from build123d import *

# Parameters (mm, degrees)
SKETCH_1_W                  = 28
SKETCH_1_H                  = 19
EXTRUDE_1_DEPTH             = 29
CUT_EXTRUDE_1_DEPTH         = 42.41557678
HOLE_WIZARD_1_D             = 10
HOLE_WIZARD_1_2_D           = 5.5
HOLE_WIZARD_1_2_CBORE_D     = 10
HOLE_WIZARD_1_2_CBORE_DEPTH = 5
CHAMFER_1_SIZE              = 5


with BuildPart() as part:
    # 草图1 → 凸台-拉伸1 (new body)
    with BuildSketch(Plane(origin=(0, 0, 0), x_dir=(1, 0, 0), z_dir=(0, 1, 0))):
        Rectangle(SKETCH_1_W, SKETCH_1_H)
    extrude(amount=-EXTRUDE_1_DEPTH)

    # 草图2 → 切除-拉伸1 (cut, through all)
    with BuildSketch(Plane(origin=(14, 0, 0), x_dir=(0, 0, -1), z_dir=(1, 0, 0))):
        with BuildLine():
            Line((9.5, -29), (-5, -29))
            Line((-5, -29), (-5, -10))
            ThreePointArc((-5, -10), (-4.121320344, -7.878679656), (-2, -7))
            Line((-2, -7), (9.5, -7))
            Line((9.5, -7), (9.5, -29))
        make_face()
    extrude(amount=-CUT_EXTRUDE_1_DEPTH, mode=Mode.SUBTRACT)

    # Hole Wizard 1 (through all)
    with Locations(Plane.XY.offset(9.5)):
        with Locations((0, -19)):
            Hole(HOLE_WIZARD_1_D / 2)

    # Hole Wizard 1 2 (through all)
    with Locations(Plane(origin=(0, -7, 0), x_dir=(-1, 0, 0), z_dir=(0, -1, 0))):
        with Locations((8, 3.5), (-8, 3.5)):
            CounterBoreHole(HOLE_WIZARD_1_2_D / 2, HOLE_WIZARD_1_2_CBORE_D / 2, HOLE_WIZARD_1_2_CBORE_DEPTH)

    # 倒角1
    chamfer_1_edges = [part.edges().sort_by_distance(p)[0] for p in [
        (-14, -29, 7.25),
        (14, -29, 7.25),
    ]]
    chamfer(chamfer_1_edges, length=CHAMFER_1_SIZE)


solid = part.part
Verification items for the finished model (mm, model axes). A direction names the side the tool comes from. Coordinates: 2 decimals unless noted, no trailing zeros. Order: outer loops, then holes, each group sorted by start corner. A loop starts at its lowest first (then second) coordinate and runs counter-clockwise, first axis right, second up. Notation, with made-up numbers: (17, 21) -> (41, 21) arc R20 ccw to (41, 31) -> close; hole circle Ø2 at (12.25, 9.25). An arc over 180 degrees is marked (long way). Put each result on its own line as item: value. Start each with the question number.
1. Material ranges on L1, parallel to Y at x = 0, z = 6.8; L2, parallel to X at y = -2.25, z = -8; L3, parallel to Z at x = -8, y = -4.65, recorded low to high. Write a range as [from, to].
2. Mould release check, pull along Z, two halves, no side actions. Record for faces 1 (the flat face through (0, -11, 9.5)), 2 (the flat face through (-11, -27, 7)), 3 (the cylindrical face through (-6.73, -0.99, -1.06)): released by +Z, released by -Z, zero draft, split by the parting line, or undercut.
3. Cross-section at D-D, the plane z = 6.5. Record the boundary of the cut face in (x, y), then the cut area to 3 significant figures.
4. Go/stop test with flat-tipped pins: pin 1 Ø5 at (x, z) = (-7.5, -5.5) entering from -Y; pin 2 Ø11.5 at (x, y) = (0, -19) entering from +Z; pin 3 Ø8 at (x, z) = (1, 0.5) entering from -Y; pin 4 Ø15 at (x, y) = (-2, -23) entering from -Z. Record where each tip stops, or that it passes through.
5. Cross-section at B-B, the plane x = -8. Record the boundary of the cut face in (y, z), then the cut area to 3 significant figures.
6. Cross-section at C-C, the plane y = -19. Record the boundary of the cut face in (x, z), then the cut area to 3 significant figures.
7. Cross-section at A-A, the plane z = -3.5. Record the boundary of the cut face in (x, y), then the cut area to 3 significant figures.
8. Access from +Z, -Z, +X, -X, +Y, -Y to the whole of each face (thin tool, end or side, straight path). Record for faces 4 (the flat face through (0, -29, 7)), 5 (the flat face through (0, -7, -4)), 6 (the flat face through (-10, -2, -1)).
Computed:
1. L1: [-29, -24], [-14, 0]
1. L2: [-14, -10.18], [-5.82, 5.82], [10.18, 14]
1. L3: [-9.5, -8.5], [1.5, 9.5]
2. face 1: released by +Z
2. face 2: zero draft
2. face 3: undercut
3. outline: (-14, -24) -> (-9, -29) -> (9, -29) -> (14, -24) -> (14, 0) -> (-14, 0) -> close; hole circle Ø10 at (0, -19)
3. area: 708 mm2
4. pin 1: y = -2
4. pin 2: z = 9.5
4. pin 3: y = -8.34
4. pin 4: z = 5
5. outline: (-29, 5) -> (-10, 5) arc R3 cw to (-7, 2) -> (-7, 1.5) -> (-2, 1.5) -> (-2, -0.75) -> (0, -0.75) -> (0, 9.5) -> (-29, 9.5) -> close; (-7, -9.5) -> (0, -9.5) -> (0, -6.25) -> (-2, -6.25) -> (-2, -8.5) -> (-7, -8.5) -> close
5. area: 173 mm2
6. outline: (-14, 5) -> (-5, 5) -> (-5, 9.5) -> (-14, 9.5) -> close; (5, 5) -> (14, 5) -> (14, 9.5) -> (5, 9.5) -> close
6. area: 81.0 mm2
7. outline: (-14, -7) -> (-13, -7) -> (-13, -2) -> (-10.75, -2) -> (-10.75, 0) -> (-14, 0) -> close; (-5.25, -2) -> (-3, -2) -> (-3, -7) -> (3, -7) -> (3, -2) -> (5.25, -2) -> (5.25, 0) -> (-5.25, 0) -> close; (10.75, -2) -> (13, -2) -> (13, -7) -> (14, -7) -> (14, 0) -> (10.75, 0) -> close
7. area: 74.0 mm2
8. face 4: +Z, -Z, +X, -X, -Y
8. face 5: -Z, +X, -X, -Y
8. face 6: -Y
